Input: part model. Units: mm. Frame: model coordinates. A direction names the side the tool comes from. Give positions to 0.01 mm unless a question says otherwise; leave off trailing zeros. Write each loop counter-clockwise with the first axis right and the second up, starting at its lowest first coordinate (ties: lowest second). Pieces come first, ordered by that corner, then holes. Notation, with made-up numbers: (-23, 24.25) - (19, 24.25) arc R26 cw to (19, 38.25) - close; hole circle Ø2 at (21, 29). An arc over 180 degrees is marked (long way). Use a Markdown table: item, result. Add a question column.
1. Section query A-A, the plane x = 16.5. Return loops of the section in (y, z).
2. Pin query (flat end, axial travel): pin 1 (5.5 mm diameter, centred on x = -1, z = 17, fed in from +Y); pin 2 (8 mm diameter, centred on x = 45.5, y = 2.5, fed in from +Z); pin 3 (4 mm diameter, centred on y = 3, z = 19.5, fed in from +X); pin 4 (0.6 mm diameter, centred on y = -9, z = 2, fed in from -X). Return the tip coordinate at first contact, or that it passes through.
3. Section query B-B, the plane z = 1.5. Return loops of the section in (x, y), plus the area to 3 significant figures.
4. Material intervals for probe 1 along X at (y, z) = (8.45, 17); probe 2 along Y at (x, z) = (1.5, 20.75); probe 3 along Y at (x, z) = (19, 6.5), sorted ascending.
5. Set-up query: faces 4 (the cylindrical face through (4.9, -8.5, 19.5)), 5 (the flat face through (18, 0, 3)), 6 (the cylindrical face through (9.719, -7.719, 22.594)), 7 (the flat face through (1, 7, 0)), 8 (the cylindrical face through (-19.163, 0.077, 6.398)). Return all of +Z, -Z, +X, -X, +Y, -Y with unobstructed straight access to the full face (end or side cutting, diameter ignored); none if empty.
6. Section query C-C, the plane x = -70.5. Return loops of the section in (y, z), plus the area to 3 significant figures.
7. Mould query, pull axis Z, two halves, no side actions, for faces 1 (the cylindrical face through (-4.9, 8.5, 19.5)), 2 (the cylindrical face through (22.293, 0.14, 5.592)), 3 (the flat face through (0, -5.5, 12)). Classes: released by +Z, released by -Z, zero draft, split by the parting line, or undercut.
```python
from build123d import *

# Parameters (mm, degrees)
BOSS_EXTRU_1_DEPTH      = 5
ESQUISSE2_R             = 5.1
ESQUISSE2_R_2           = 2.1
ENL_V_MAT_EXTRU_1_DEPTH = 91.691785736
ESQUISSE3_W             = 24
ESQUISSE3_H             = 20
BOSS_EXTRU_2_DEPTH      = 20
CHANFREIN1_SIZE         = 10
ESQUISSE4_W             = 36
ESQUISSE4_H             = 11
ENL_V_MAT_EXTRU_2_DEPTH = 20
ESQUISSE5_R             = 2.1
ENL_V_MAT_EXTRU_3_DEPTH = 96.524865873
CONG_1_R                = 8
ESQUISSE6_R             = 5.5
ENL_V_MAT_EXTRU_4_DEPTH = 2
CHANFREIN2_SIZE         = 1
CONG_4_R                = 2
ENL_V_START             = -2
ESQUISSE7_R             = 5.5
ENL_V_MAT_EXTRU_5_DEPTH = 2
CHANFREIN3_SIZE         = 1
ESQUISSE8_W             = 36
ESQUISSE8_H             = 11
ENL_V_MAT_EXTRU_6_DEPTH = 93.736184955
ESQUISSE9_W             = 2
ESQUISSE9_H             = 5
ENL_V_MAT_EXTRU_7_DEPTH = 2


with BuildPart() as part:
    # Esquisse1 → Boss.-Extru.1 (new body)
    with BuildSketch(Plane.XY):
        with BuildLine():
            Line((-80, 10), (80, 10))
            ThreePointArc((80, 10), (90, 0), (80, -10))
            Line((80, -10), (-80, -10))
            ThreePointArc((-80, -10), (-90, 0), (-80, 10))
        make_face()
    extrude(amount=BOSS_EXTRU_1_DEPTH)

    # Esquisse2 → Enlèv. mat.-Extru.1 (cut, through all)
    with BuildSketch(Plane.XY.offset(5)):
        with Locations((-80, 0)):
            Circle(ESQUISSE2_R)
        with Locations((80, 0)):
            Circle(ESQUISSE2_R)
        with Locations((-50, 0)):
            Circle(ESQUISSE2_R_2)
        with Locations((50, 0)):
            Circle(ESQUISSE2_R_2)
    extrude(amount=-ENL_V_MAT_EXTRU_1_DEPTH, mode=Mode.SUBTRACT)

    # Esquisse3 → Boss.-Extru.2 (add)
    with BuildSketch(Plane.XY.offset(5)):
        Rectangle(ESQUISSE3_W, ESQUISSE3_H)
    extrude(amount=BOSS_EXTRU_2_DEPTH)

    # Chanfrein1
    chanfrein1_edges = [part.edges().sort_by_distance(p)[0] for p in [
        (12, 0, 5),
        (-12, 0, 5),
    ]]
    chamfer(chanfrein1_edges, length=CHANFREIN1_SIZE)

    # Esquisse4 → Enlèv. mat.-Extru.2 (cut)
    with BuildSketch(Plane.XY.offset(25)):
        Rectangle(ESQUISSE4_W, ESQUISSE4_H)
    extrude(amount=-ENL_V_MAT_EXTRU_2_DEPTH, mode=Mode.SUBTRACT)

    # Esquisse5 → Enlèv. mat.-Extru.3 (cut, through all)
    with BuildSketch(Plane(origin=(0, 10, 0), x_dir=(1, 0, 0), z_dir=(0, 1, 0))):
        with Locations(Location((0, -17, 0), (0, 0, 270))):
            Circle(ESQUISSE5_R)
    extrude(amount=-ENL_V_MAT_EXTRU_3_DEPTH, mode=Mode.SUBTRACT)

    # Congé1
    cong_1_edges = [part.edges().sort_by_distance(p)[0] for p in [
        (-22, 0, 5),
        (-12, -7.75, 25),
        (12, -7.75, 25),
        (22, 0, 5),
        (-12, 7.75, 25),
        (12, 7.75, 25),
    ]]
    fillet(cong_1_edges, radius=CONG_1_R)

    # Esquisse6 → Enlèv. mat.-Extru.4 (cut)
    with BuildSketch(Plane(origin=(0, 10, 0), x_dir=(1, 0, 0), z_dir=(0, 1, 0))):
        with Locations(Location((0, -17, 0), (0, 0, 270))):
            Circle(ESQUISSE6_R)
    extrude(amount=-ENL_V_MAT_EXTRU_4_DEPTH, mode=Mode.SUBTRACT)

    # Chanfrein2
    chanfrein2_edges = [part.edges().sort_by_distance(p)[0] for p in [
        (0, 10, 11.5),
    ]]
    chamfer(chanfrein2_edges, length=CHANFREIN2_SIZE)

    # Congé4
    # the kernel refuses this fillet: 2 mm, written as the material it takes off along each edge
    with BuildSketch(Plane(origin=(18, -5.5, 9), x_dir=(0.7394878589424565, 0, -0.6731698942144558), z_dir=(0, 1, 0)), Plane(origin=(-18, 5.5, 9), x_dir=(-0.7394878589424565, 0, -0.6731698942144557), z_dir=(0, -1, 0))) as cong_4_piece_1:
        with BuildLine():
            CenterArc((4.431818389, 1.970329953), CONG_4_R, 150.40864019, 109.709922664)
            Line((2.692679577, 2.957951436), (2.518765696, 3.056713584))
            ThreePointArc((2.518765696, 3.056713584), (1.198442217, 1.613609697), (-0.147897572, 0.134633979))
            Line((-0.147897572, 0.134633979), (0.009378777, -0.199779975))
            ThreePointArc((0.009378777, -0.199779975), (2.349946778, -0.089900774), (4.054276537, -0.197032995))
            Line((4.054276537, -0.197032995), (4.088598523, 0))
        make_face()
    extrude(amount=11, mode=Mode.SUBTRACT)

    # Esquisse7 → Enlèv. mat.-Extru.5 (cut)
    with BuildSketch(Plane.XZ.offset(10).offset(ENL_V_START)):
        with Locations(Location((0, 17, 0), (0, 0, 90))):
            Circle(ESQUISSE7_R)
    extrude(amount=ENL_V_MAT_EXTRU_5_DEPTH, mode=Mode.SUBTRACT)

    # Chanfrein3
    chanfrein3_edges = [part.edges().sort_by_distance(p)[0] for p in [
        (0, -10, 11.5),
    ]]
    chamfer(chanfrein3_edges, length=CHANFREIN3_SIZE)

    # Esquisse8 → Enlèv. mat.-Extru.6 (cut, through all)
    with BuildSketch(Plane.XY.offset(5)):
        Rectangle(ESQUISSE8_W, ESQUISSE8_H)
    extrude(amount=-ENL_V_MAT_EXTRU_6_DEPTH, mode=Mode.SUBTRACT)

    # Esquisse9 → Enlèv. mat.-Extru.7 (cut)
    with BuildSketch(Plane.XZ.offset(10)):
        with Locations((0, 2.5)):
            Rectangle(ESQUISSE9_W, ESQUISSE9_H)
    extrude(amount=-ENL_V_MAT_EXTRU_7_DEPTH, mode=Mode.SUBTRACT)


solid = part.part
```
Result sheet:
| question | item | result |
|---|---|---|
| 1 | outline | (-10, 0) - (-5.5, 0) - (-5.5, 10.5) - (-10, 10.5) - close; (5.5, 0) - (10, 0) - (10, 10.5) - (5.5, 10.5) - close |
| 2 | pin 1 | stops at y = 8 |
| 2 | pin 2 | stops at z = 5 |
| 2 | pin 3 | passes through |
| 2 | pin 4 | stops at x = -84.93 |
| 3 | outline | (-80, -10) - (-1, -10) - (-1, -8) - (1, -8) - (1, -10) - (80, -10) arc R10 ccw to (80, 10) - (-80, 10) arc R10 ccw to start; hole circle Ø10.2 at (-80, 0); hole circle Ø4.2 at (-50, 0); hole (-18, -5.5) - (18, -5.5) - (18, 5.5) - (-18, 5.5) - close; hole circle Ø4.2 at (50, 0); hole circle Ø10.2 at (80, 0) |
| 3 | area | 2,920 mm² |
| 4 | probe 1 | x = -12 to -5.5, 5.5 to 12 |
| 4 | probe 2 | y = -8 to -5.5, 5.5 to 8 |
| 4 | probe 3 | y = -10 to -5.5, 5.5 to 10 |
| 5 | face 4 | -Y |
| 5 | face 5 | +Z, -Z |
| 5 | face 6 | +Z, +X, +Y, -Y |
| 5 | face 7 | -Z, +X, -X, +Y, -Y |
| 5 | face 8 | +Z |
| 6 | outline | (-10, 0) - (10, 0) - (10, 5) - (-10, 5) - close |
| 6 | area | 100 mm² |
| 7 | face 1 | undercut |
| 7 | face 2 | released by +Z |
| 7 | face 3 | zero draft |
